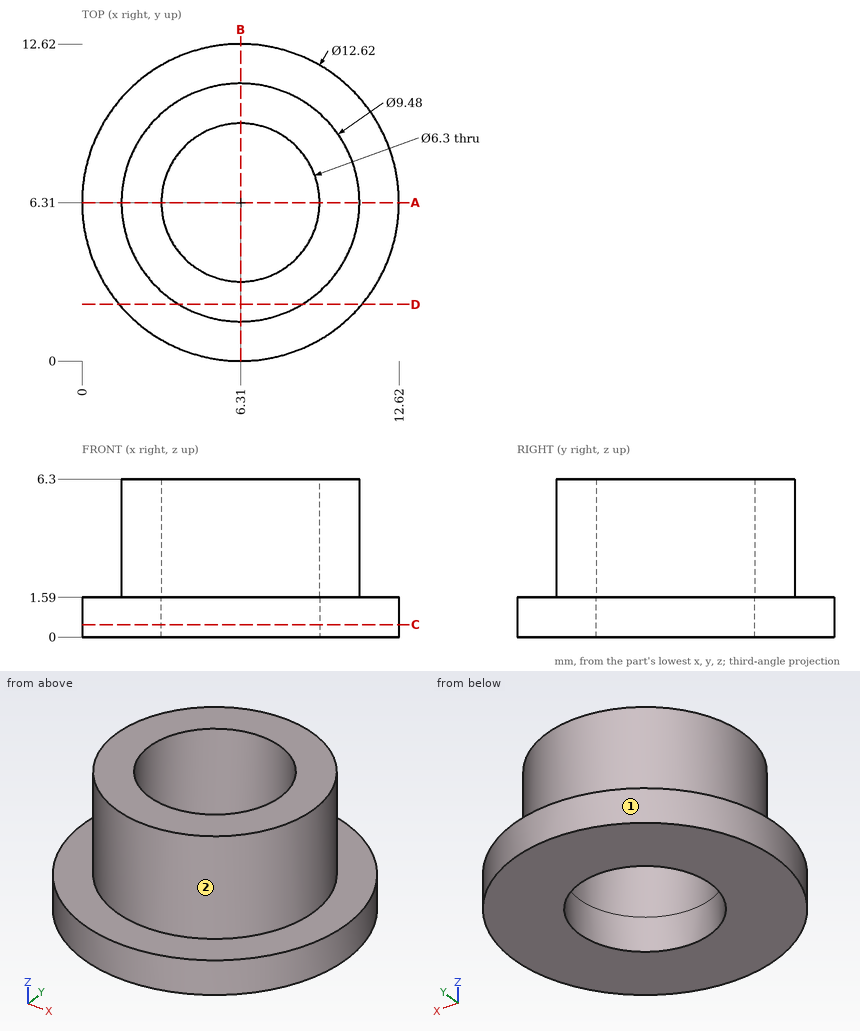
Answer from the drawing. Dimensions are ordinates in mm from the lowest x, y and z of the part. A direction names the side the tool comes from. Round coordinates to 2 decimals unless told otherwise and drop trailing zeros. Write each loop counter-clockwise with the first axis right and the second up, starting at its lowest first coordinate (ties: lowest second). Pieces come first, ordered by that corner, then holes. Notation, with made-up numbers: M 89,26.5 L 112,26.5 A14 cw 112,44.5 Z; hole C 37.25,44.25 d4. An arc over 180 degrees is marked long. Write each question's results on one line, items separated by ' | '. Start each with the question number.
Item 1: Find section D-D on y = 2.25. Write down the section's boundary in (x, z).
Item 2: Straight lines are drawn through the part: probe 1 along Y at (x, z) = (6.31, 3.25); probe 2 along Y at (x, z) = (6.31, 0.45); probe 3 along Z at (x, y) = (2.75, 2.25). For each, find the intervals that lie inside material, in ascending order.
Item 3: Given pin 1 Ø6 at (x, y) = (6.5, 6) entering from +Z; pin 2 Ø1 at (x, z) = (3.5, 3.5) entering from -Y; pin 3 Ø1 at (x, y) = (10.5, 10) entering from +Z; pin 4 Ø2 at (x, z) = (9, 1) entering from -Y, each flat-ended and moving along its own axis, determine where each tip first touches the part or whether it passes through.
Item 4: Find section C-C on z = 0.5. Write down the section's boundary in (x, y), and give its area (3 significant figures).
Item 5: Which of the six approach directions +Z, -Z, +X, -X, +Y, -Y give full straight-line access (tool end or side, diameter ignored) to the marked faces 1 and 2?
Item 6: Find section A-A on y = 6.31. Write down the section's boundary in (x, z), and give its area (3 significant figures).
Answer block:
1) outline: M 1.48,0 L 11.14,0 L 11.14,1.59 L 8.76,1.59 L 8.76,6.3 L 3.86,6.3 L 3.86,1.59 L 1.48,1.59 Z
2) probe 1: y = 1.57 to 3.16, 9.46 to 11.05 | probe 2: y = 0 to 3.16, 9.46 to 12.62 | probe 3: z = 0 to 1.59
3) pin 1: stops at z = 6.3 | pin 2: stops at y = 2.17 | pin 3: stops at z = 1.59 | pin 4: stops at y = 0.23
4) outline: C 6.31,6.31 d12.62; hole C 6.31,6.31 d6.3 | area: 93.9 mm²
5) face 1: +Z, -Z | face 2: +Z
6) outline: M 0,0 L 3.16,0 L 3.16,6.3 L 1.57,6.3 L 1.57,1.59 L 0,1.59 Z; M 9.46,0 L 12.62,0 L 12.62,1.59 L 11.05,1.59 L 11.05,6.3 L 9.46,6.3 Z | area: 25.0 mm²
